Solid Edge part; units mm, degrees
sketch "Sketch1" plane through (0, 0, 0) normal (0, 0, 1) x (1, 0, 0)
  line L0 (-3.25, -3.25) -> (3.25, -3.25)
  line L1 (3.25, -3.25) -> (3.25, 3.25)
  line L2 (3.25, 3.25) -> (-3.25, 3.25)
  line L3 (-3.25, 3.25) -> (-3.25, -3.25)
  dimension "D1" = 3.25
extrude "Protrusion1" add sketch "Sketch1" along normal blind 3
sketch "Sketch2" plane through (0, 0, 3) normal (0, 0, 1) x (1, 0, 0)
  circle A0 centre (0, 0) radius 1.5
extrude "Ajout_matière_2" add sketch "Sketch2" along normal blind 3
properties material "Acier"
For this review, take the finished solid that the model builds, in its own axes (mm). A direction names the side the tool comes from. Round coordinates to 2 decimals unless told otherwise and drop trailing zeros. Order: outer loops, then holes, each group sorted by start corner. A loop starts at its lowest first (then second) coordinate and runs counter-clockwise, first axis right, second up. Notation, with made-up numbers: M 45.5,-28.5 L 73.5,-28.5 A23 ccw 73.5,3.5 Z; hole C 65.5,81.25 d5. An arc over 180 degrees is marked long. Use a Markdown table: item, result. Add a question column.
Item 1: Insertion check: pin 1 (1 mm diameter, centred on x = -1.5, y = -2, fed in from +Z). The pin has a flat end and moves straight along its axis. Give the tip position at first contact, or say it passes through.
Item 2: Add section B-B, the plane y = 1. Give the boundary of the cut face in (x, z), then the cut area to 3 significant figures.
Item 3: Tool access review of faces 1 (the cylindrical face through (-1.5, -0.07, 4.48)), 2 (the flat face through (3.25, 0, 1)): name each direction out of +Z, -Z, +X, -X, +Y, -Y from which nothing blocks a thin tool from reaching the whole face with its end or side.
Item 4: To check wall thickness, follow line 1 along Z through (x, y) = (1.5, -2.75); line 2 along X through (y, z) = (-1.25, 4.6); line 3 along X through (y, z) = (-0.25, 5.7). State the ranges of each line that lie inside material, in increasing order.
Item 5: Add section C-C, the plane z = 3.3. Give the boundary of the cut face in (x, y).
Item 6: Add section A-A, the plane x = 0. Give the boundary of the cut face in (y, z), then the cut area to 3 significant figures.
Item 7: Add section D-D, the plane x = -1.75. Give the boundary of the cut face in (y, z), then the cut area to 3 significant figures.
Geometry results:
| question | item | result |
|---|---|---|
| 1 | pin 1 | stops at z = 3 |
| 2 | outline | M -3.25,0 L 3.25,0 L 3.25,3 L 1.12,3 L 1.12,6 L -1.12,6 L -1.12,3 L -3.25,3 Z |
| 2 | area | 26.2 mm² |
| 3 | face 1 | +Z |
| 3 | face 2 | +Z, -Z, +X, +Y, -Y |
| 4 | line 1 | z = 0 to 3 |
| 4 | line 2 | x = -0.83 to 0.83 |
| 4 | line 3 | x = -1.48 to 1.48 |
| 5 | outline | C 0,0 d3 |
| 6 | outline | M -3.25,0 L 3.25,0 L 3.25,3 L 1.5,3 L 1.5,6 L -1.5,6 L -1.5,3 L -3.25,3 Z |
| 6 | area | 28.5 mm² |
| 7 | outline | M -3.25,0 L 3.25,0 L 3.25,3 L -3.25,3 Z |
| 7 | area | 19.5 mm² |
